```python
from build123d import *

# Parameters (mm, degrees)
SKETCH1_W                   = 107.95
SKETCH1_H                   = 81.28
BOSS_EXTRUDE1_DEPTH         = 2.54
M5_CLEARANCE_HOLE1_D        = 5.8
F_97_0_981_DIAMETER_HOLE1_D = 24.9174
FILLET1_R                   = 6.35


with BuildPart() as part:
    # Sketch1 → Boss-Extrude1 (new body)
    with BuildSketch(Plane(origin=(0, 0, 0), x_dir=(1, 0, 0), z_dir=(0, 1, 0))):
        with Locations((53.975, 40.64)):
            Rectangle(SKETCH1_W, SKETCH1_H)
    extrude(amount=BOSS_EXTRUDE1_DEPTH)

    # M5 Clearance Hole1 (through all)
    with Locations(Plane(origin=(0, 2.54, 0), x_dir=(1, 0, 0), z_dir=(0, 1, 0))):
        with Locations((15.875, 53.34), (41.275, 53.34), (41.275, 27.94), (15.875, 27.94), (10.541, 40.64)):
            Hole(M5_CLEARANCE_HOLE1_D / 2)

    # #97 (0.981) Diameter Hole1 (through all)
    with Locations(Plane(origin=(0, 2.54, 0), x_dir=(1, 0, 0), z_dir=(0, 1, 0))):
        with Locations((28.575, 40.64)):
            Hole(F_97_0_981_DIAMETER_HOLE1_D / 2)

    # Fillet1
    fillet1_edges = [part.edges().sort_by_distance(p)[0] for p in [
        (0, 1.27, -81.28),
        (107.95, 1.27, -81.28),
        (107.95, 1.27, 0),
        (0, 1.27, 0),
    ]]
    fillet(fillet1_edges, radius=FILLET1_R)


solid = part.part
```
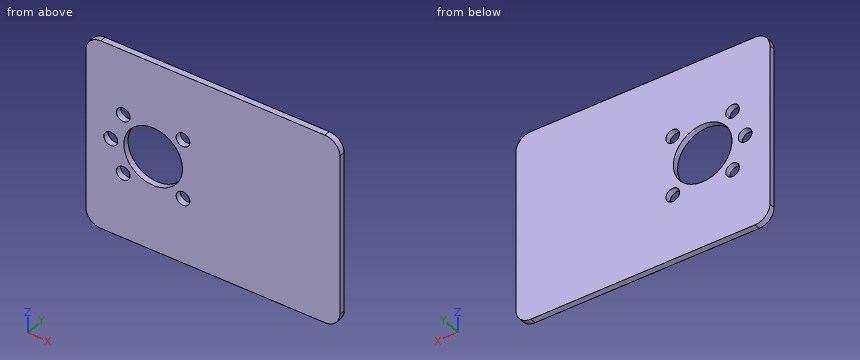
Model file for the job. Use its own axes, mm. Coordinates: 2 decimals unless noted, no trailing zeros. Order: outer loops, then holes, each group sorted by start corner. A loop starts at its lowest first (then second) coordinate and runs counter-clockwise, first axis right, second up. Notation, with made-up numbers: (28, 57) -> (84, 57) arc R26 cw to (84, 80) -> close; hole circle Ø10 at (-13, -9). An arc over 180 degrees is marked (long way). Answer as a JSON object with one key per item and string values. Group by question number.
1) Cut at B-B, the plane z = -40.64. Write the cut outline in (x, y).
2) Drill centre lines: L1, parallel to X at y = 1.85, z = -27.94 (3 decimals); L2, parallel to Z at x = 10.5, y = 1.95; L3, parallel to X at y = 1.45, z = -40. Where is each one in solid material? Low to high.
3) Flat gauge pin, fed straight in: pin 1 (8 mm diameter, centred on x = 35, z = -31.5, fed in from -Y). Where does the tip first touch, or does it go through?
4) Cut at A-A, the plane y = 1.4. Write the cut outline in (x, z) (3 decimals), then the cut area to 3 significant figures.
5) Cut at C-C, the plane x = 28.5. Write the cut outline in (y, z), then the cut area to 3 significant figures.
Check values:
{
 "1": {"outline": "(0, 0) -> (7.64, 0) -> (7.64, 2.54) -> (0, 2.54) -> close; (13.44, 0) -> (16.12, 0) -> (16.12, 2.54) -> (13.44, 2.54) -> close; (41.03, 0) -> (107.95, 0) -> (107.95, 2.54) -> (41.03, 2.54) -> close"},
 "2": {"L1": "x = 0 to 12.975, 18.775 to 38.375, 44.175 to 107.95", "L2": "z = -81.28 to -43.54, -37.74 to 0", "L3": "x = 0 to 7.71, 13.37 to 16.13, 41.02 to 107.95"},
 "3": {"pin 1": "stops at y = 0"},
 "4": {"outline": "(0, -74.93) arc R6.35 ccw to (6.35, -81.28) -> (101.6, -81.28) arc R6.35 ccw to (107.95, -74.93) -> (107.95, -6.35) arc R6.35 ccw to (101.6, 0) -> (6.35, 0) arc R6.35 ccw to (0, -6.35) -> close; hole circle Ø5.8 at (10.541, -40.64); hole circle Ø5.8 at (15.875, -53.34); hole circle Ø5.8 at (15.875, -27.94); hole circle Ø24.917 at (28.575, -40.64); hole circle Ø5.8 at (41.275, -53.34); hole circle Ø5.8 at (41.275, -27.94)", "area": "8,120 mm²"},
 "5": {"outline": "(0, -81.28) -> (2.54, -81.28) -> (2.54, -53.1) -> (0, -53.1) -> close; (0, -28.18) -> (2.54, -28.18) -> (2.54, 0) -> (0, 0) -> close", "area": "143 mm²"}
}
